For this review, take the finished solid that the model builds, in its own axes (mm). Face numbers are marked on the shaded views. A direction names the side the tool comes from. Coordinates: 2 decimals unless noted, no trailing zeros. Write each loop counter-clockwise with the first axis right and the second up, starting at its lowest first coordinate (ties: lowest second). Pieces come first, ordered by that corner, then holes. Notation, with made-up numbers: (57, -7) - (78, -7) arc R23 ccw to (78, 5) - close; hole circle Ø3 at (33, 2). An arc over 180 degrees is marked (long way). Use one line per item in the form item = value. Start each with the question number.
1) Insertion check: P1, Ø10, axis at x = -1, z = -5, coming from the +Y side; P2, Ø18, axis at x = 4, z = 3.5, coming from the +Y side. Each pin has a flat end and moves straight along its axis. Give the tip position at first contact, or say it passes through.
2) Tool access review of the marked faces 5 and 6: name each direction out of +Z, -Z, +X, -X, +Y, -Y from which nothing blocks a thin tool from reaching the whole face with its end or side.
3) We need section A-A (x = 0). Give the boundary of the cut face in (y, z) (3 decimals), plus the area to 3 significant figures.
4) Mouldability with a two-part tool opening along Z and no side actions: class the marked faces 1, 2, 3 and 4 as pulls with the +Z half, pulls with the -Z half, needs draft (parallel to the pull), parting line crosses it, or undercut.
5) We need section D-D (z = 9). Give the boundary of the cut face in (x, y).
6) For L1, parallel to Z at x = 0, y = -1.3; L2, parallel to X at y = -0.25, z = 10; L3, parallel to X at y = -2.75, z = -10, list the stretches that pass through material, from the lowest coordinate up. Write a range as from..to.
7) We need section C-C (y = -0.9). Give the boundary of the cut face in (x, z).
8) We need section B-B (z = 0). Give the boundary of the cut face in (x, y) (3 decimals), plus the area to 3 significant figures.
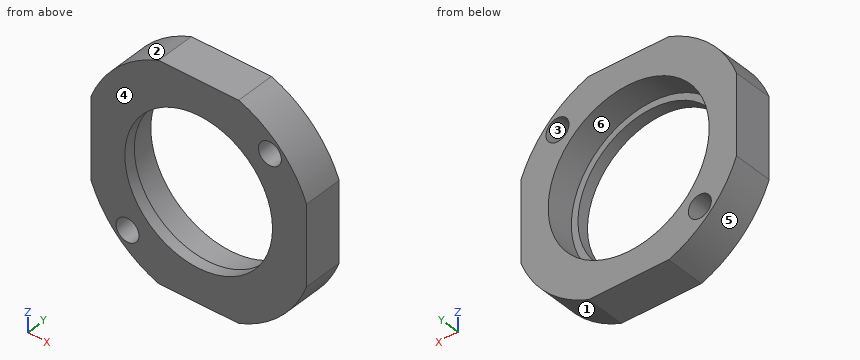
```python
from build123d import *

# Parameters (mm, degrees)
BOSS_EXTRUDE1_DEPTH = 5.5
SKETCH2_R           = 11.2
CUT_EXTRUDE1_DEPTH  = 22.914607001
SKETCH3_R           = 1.6
CUT_EXTRUDE2_DEPTH  = 22.914607001
BOSS_EXTRUDE2_START = -1.6
SKETCH4_R           = 11.2
SKETCH4_R_2         = 10.275
BOSS_EXTRUDE2_DEPTH = 1.6


with BuildPart() as part:
    # Sketch1 → Boss-Extrude1 (new body)
    with BuildSketch(Plane(origin=(0, 0, 0), x_dir=(1, 0, 0), z_dir=(0, 1, 0))):
        with BuildLine():
            ThreePointArc((15, 5.567764363), (11.313708499, 11.313708499), (5.567764363, 15))
            Line((5.567764363, 15), (-5.567764363, 15))
            ThreePointArc((-5.567764363, 15), (-11.313708499, 11.313708499), (-15, 5.567764363))
            Line((-15, 5.567764363), (-15, -5.567764363))
            ThreePointArc((-15, -5.567764363), (-11.313708499, -11.313708499), (-5.567764363, -15))
            Line((-5.567764363, -15), (5.567764363, -15))
            ThreePointArc((5.567764363, -15), (11.313708499, -11.313708499), (15, -5.567764363))
            Line((15, -5.567764363), (15, 5.567764363))
        make_face()
    extrude(amount=-BOSS_EXTRUDE1_DEPTH)

    # Sketch2 → Cut-Extrude1 (cut, through all)
    with BuildSketch(Plane(origin=(0, 0, 0), x_dir=(1, 0, 0), z_dir=(0, 1, 0))):
        with Locations(Location((0, 0, 0), (0, 0, 270))):
            Circle(SKETCH2_R)
    extrude(amount=-CUT_EXTRUDE1_DEPTH, mode=Mode.SUBTRACT)

    # Sketch3 → Cut-Extrude2 (cut, through all)
    with BuildSketch(Plane(origin=(0, 0, 0), x_dir=(1, 0, 0), z_dir=(0, 1, 0))):
        with Locations(Location((-9.899494937, 9.899494937, 0), (0, 0, 270))):
            Circle(SKETCH3_R)
        with Locations(Location((9.899494937, -9.899494937, 0), (0, 0, 270))):
            Circle(SKETCH3_R)
    extrude(amount=-CUT_EXTRUDE2_DEPTH, mode=Mode.SUBTRACT)

    # Sketch4 → Boss-Extrude2 (add)
    with BuildSketch(Plane.XZ.offset(5.5).offset(BOSS_EXTRUDE2_START)):
        with Locations(Location((0, 0, 0), (0, 0, 90))):
            Circle(SKETCH4_R)
        with Locations(Location((0, 0, 0), (0, 0, 270))):
            Circle(SKETCH4_R_2, mode=Mode.SUBTRACT)
    extrude(amount=BOSS_EXTRUDE2_DEPTH)


solid = part.part
```
Determined:
q1.P1 = through
q1.P2 = 0
q2.face_5 = -Z, -X, +Y, -Y
q2.face_6 = +Y
q3.outline = (-5.5, -15) - (0, -15) - (0, -11.2) - (-3.9, -11.2) - (-3.9, -10.275) - (-5.5, -10.275) - close; (-5.5, 10.275) - (-3.9, 10.275) - (-3.9, 11.2) - (0, 11.2) - (0, 15) - (-5.5, 15) - close
q3.area = 44.8 mm²
q4.face_1 = pulls with the -Z half
q4.face_2 = pulls with the +Z half
q4.face_3 = undercut
q4.face_4 = needs draft
q5.outline = (-13.23, -5.5) - (-4.96, -5.5) - (-4.96, -3.9) - (-6.67, -3.9) - (-6.67, 0) - (-13.23, 0) - close; (4.96, -5.5) - (8.58, -5.5) - (8.58, 0) - (6.67, 0) - (6.67, -3.9) - (4.96, -3.9) - close; (11.22, -5.5) - (13.23, -5.5) - (13.23, 0) - (11.22, 0) - close
q6.L1 = -15..-11.2, 11.2..15
q6.L2 = -12.49..-5.04, 5.04..8.3, 11.5..12.49
q6.L3 = -12.49..-11.5, -8.3..-5.04, 5.04..12.49
q7.outline = (-15, -5.57) arc R16 ccw to (-5.57, -15) - (5.57, -15) arc R16 ccw to (15, -5.57) - (15, 5.57) arc R16 ccw to (5.57, 15) - (-5.57, 15) arc R16 ccw to (-15, 5.57) - close; hole circle Ø3.2 at (-9.9, -9.9); hole circle Ø22.4 at (0, 0); hole circle Ø3.2 at (9.9, 9.9)
q8.outline = (-15, -5.5) - (-10.275, -5.5) - (-10.275, -3.9) - (-11.2, -3.9) - (-11.2, 0) - (-15, 0) - close; (10.275, -5.5) - (15, -5.5) - (15, 0) - (11.2, 0) - (11.2, -3.9) - (10.275, -3.9) - close
q8.area = 44.8 mm²
